Build history of the part. All positions in model axes, mm. A direction names the side the tool comes from. Give positions to 0.01 mm unless a question says otherwise; leave off trailing zeros. Order: outer loops, then holes, each group sorted by start corner. A loop starts at its lowest first (then second) coordinate and runs counter-clockwise, first axis right, second up. Notation, with made-up numbers: (-22, 8.25) -> (30, 8.25) arc R28 cw to (30, 43.25) -> close; hole circle Ø9 at (3.5, 10.25). An arc over 180 degrees is marked (long way). One line per item, written item: value. Start each with the question number.
(1) Saw through at A-A on z = -13.5. Give the cut face in (x, y), plus the area to 3 significant figures.
(2) Saw through at B-B on y = 17. Give the cut face in (x, z), plus the area to 3 significant figures.
(3) Saw through at D-D on z = 0. Give the cut face in (x, y).
(4) Which spindle directions (+Z, -Z, +X, -X, +Y, -Y) get a long thin tool onto all of the face, cutting with end or side? Do faces 1 (the flat face through (27.5, 21.3, -5)), 2 (the flat face through (14, 8, -15)), 3 (the flat face through (28, 15, -18)). Say none if no direction does.
(5) Two-plate mould, pull along Y, no slides. Class faces 4 (the flat face through (16, 5, -12)), 5 (the flat face through (18, 23, -18)), 6 (the flat face through (16, 3, -14)), 7 (the flat face through (10, 25, -12)): +Y half, -Y half, draft (parallel to the pull), parting line (faces both ways), or undercut.
(6) Saw through at C-C on x = 16. Give the cut face in (y, z).
(7) Pin check, flat tips, straight feed: pin 1 (6 mm diameter, centred on x = 14.5, y = 18.5, fed in from -Z); pin 2 (1 mm diameter, centred on x = 27, y = 20.5, fed in from -Z). Stop position of each tip, or through.
(8) Probe line 1 (Z direction, x = -1, y = 18); line 2 (Z direction, x = 4.5, y = 11); line 3 (Z direction, x = 20, y = 31.55). List the from-to ranges inside material, lowest first.
Autodesk Inventor part; units mm, degrees
ref_plane "YZ Plane" through (0, 0, 0) normal (1, 0, 0) x (0, 1, 0)
ref_plane "XZ Plane" through (0, 0, 0) normal (0, 1, 0) x (-1, 0, 0)
ref_plane "XY Plane" through (0, 0, 0) normal (0, 0, 1) x (1, 0, 0)
ref_plane "Work Plane13" through (0, 3, 0) normal (0, 1, 0) x (1, 0, 0)
sketch "Sketch45" plane through (0, 3, 0) normal (0, 1, 0) x (1, 0, 0)
  line L0 (35, -20) -> (-3, -20)
  line L1 (-3, -20) -> (-3, 20)
  line L2 (-3, 20) -> (35, 20)
  line L3 (35, 20) -> (35, -20)
  point P0 (0, 0)
  dimension "d142" = 38
  dimension "d143" = 40
extrude "Extrusion34" add sketch "Sketch45" along normal blind 30
sketch "Sketch46" plane through (0, 33, 0) normal (0, 1, 0) x (1, 0, 0)
  point P0 (0, 0)
ref_plane "Work Plane11" through (0, 0, 0) normal (0, -1, 0) x (1, 0, 0)
sketch "Sketch47" plane through (0, 0, 0) normal (0, -1, 0) x (1, 0, 0)
  circle A0 centre (16, 0) radius 18
  point P0 (0, 0)
  dimension "d146" = 36
extrude "Extrusion35" cut sketch "Sketch47" against normal blind 30 draft -15
sketch "Sketch48" plane through (0, 33, 0) normal (0, 1, 0) x (1, 0, 0)
  point P0 (0, 0)
sketch "Sketch49" plane through (0, 33, 0) normal (0, 1, 0) x (1, 0, 0)
  circle A0 centre (20, 0) radius 1
  point P0 (0, 0)
  dimension "d149" = 2
extrude "Extrusion36" cut sketch "Sketch49" against normal through all
ref_plane "Work Plane7" through (35, 3, -20) normal (0, 0, -1) x (-1, 0, 0)
sketch "Sketch58" plane through (35, 3, -20) normal (0, 0, -1) x (-1, 0, 0)
  line L0 (7, 20) -> (27, 20)
  line L1 (27, 20) -> (27, 5)
  line L2 (27, 5) -> (7, 5)
  line L3 (7, 5) -> (7, 20)
  point P0 (35, -3)
  dimension "d156" = 20
  dimension "d157" = 15
extrude "Extrusion38" cut sketch "Sketch58" against normal blind 15
ref_plane "Work Plane4" through (-3, 3, -20) normal (-1, 0, 0) x (0, 0, 1)
sketch "Sketch59" plane through (-3, 3, -20) normal (-1, 0, 0) x (0, 0, 1)
  line L0 (4.8, 25) -> (8, 25)
  line L1 (8, 25) -> (8, 5)
  line L2 (8, 5) -> (4.8, 5)
  line L3 (4.8, 5) -> (4.8, 25)
  point P0 (20, -3)
  dimension "d160" = 3.2
  dimension "d161" = 20
extrude "Extrusion39" cut sketch "Sketch59" against normal blind 35
ref_plane "Work Plane1" through (0, 3, 0) normal (0, 1, 0) x (1, 0, 0)
ref_plane "Work Plane6" through (0, 23, 0) normal (0, 1, 0) x (1, 0, 0)
sketch "Sketch62" plane through (-3, 3, -20) normal (-1, 0, 0) x (0, 0, 1)
  circle A0 centre (20, 15) radius 3
  point P0 (20, -3)
  dimension "d172" = 6
extrude "Extrusion42" cut sketch "Sketch62" against normal through all
sketch "Sketch65" plane through (0, 3, 0) normal (0, -1, 0) x (1, 0, 0)
  line L0 (-3, -12) -> (32, -12)
  line L1 (28, -20) -> (28, -15.2)
  line L2 (3.5815, -12) -> (28, -12)
  line L3 (28, -12) -> (28, -17.2375)
  line L4 (28, -17.2375) -> (3.5815, -17.2375)
  line L5 (3.5815, -17.2375) -> (3.5815, -12)
  point P0 (0, 0)
extrude "Extrusion44" add sketch "Sketch65" against normal blind 5
properties part number "liquid port_only_v06"
Results below:
1. outline: (-3, 3) -> (35, 3) -> (35, 33) -> (-3, 33) -> (-3, 28) -> (32, 28) -> (32, 8) -> (-3, 8) -> close
1. area: 440 mm²
2. outline: (-3, -20) -> (8, -20) -> (8, -15.2) -> (-3, -15.2) -> close; (-3, -12) -> (8, -12) -> (8, -10.81) arc R13.44 cw to (2.86, -2.83) -> (-3, -2.83) -> close; (-3, 2.83) -> (2.86, 2.83) arc R13.44 cw to (29.14, 2.83) -> (35, 2.83) -> (35, 20) -> (-3, 20) -> close; (28, -20) -> (35, -20) -> (35, -2.83) -> (29.14, -2.83) arc R13.44 cw to (28, -6.06) -> (28, -12) -> (32, -12) -> (32, -15.2) -> (28, -15.2) -> close
2. area: 677 mm²
3. outline: (-3, 3) -> (-1.2, 3) -> (2.02, 15) -> (-3, 15) -> close; (-3, 21) -> (3.63, 21) -> (6.04, 30) -> (19, 30) -> (19, 33) -> (-3, 33) -> close; (21, 30) -> (25.96, 30) -> (28.37, 21) -> (35, 21) -> (35, 33) -> (21, 33) -> close; (29.98, 15) -> (33.2, 3) -> (35, 3) -> (35, 15) -> close
4. face 1: -Z, -Y
4. face 2: none
4. face 3: -Z
5. face 4: draft
5. face 5: undercut
5. face 6: -Y half
5. face 7: undercut
6. outline: (3, -20) -> (8, -20) -> (8, -12) -> (3, -12) -> close; (3, 17.2) -> (30, 9.96) -> (30, -9.96) -> (23, -11.84) -> (23, -12) -> (28, -12) -> (28, -15.2) -> (23, -15.2) -> (23, -20) -> (33, -20) -> (33, 20) -> (3, 20) -> close
7. pin 1: stops at z = 11.94
7. pin 2: stops at z = -5
8. line 1: z = -20 to -15.2, -12 to -3, 3 to 20
8. line 2: z = -20 to -15.2, -12 to -9.71, 9.71 to 20
8. line 3: z = -20 to -1, 1 to 20
